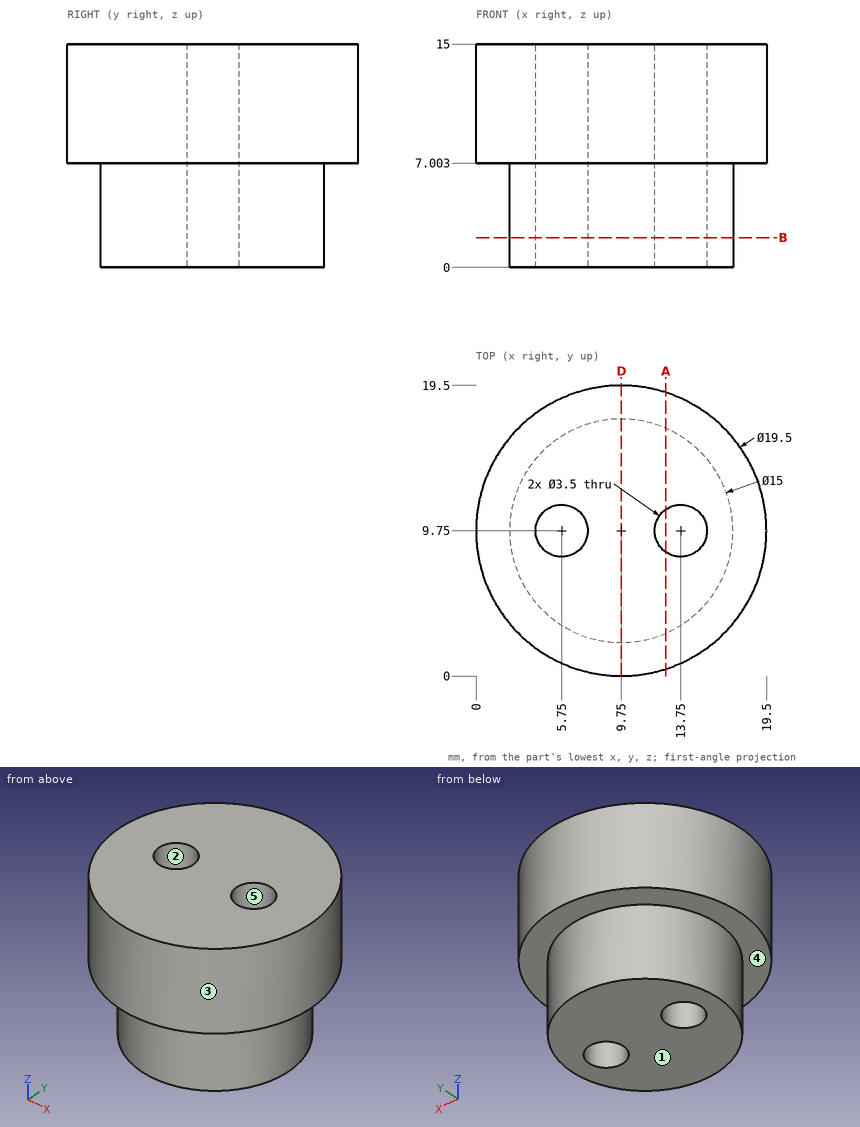
Here's the drawing with two shaded views (mm, measured from the low corner). I have some questions. A direction names the side the tool comes from. Round coordinates to 2 decimals unless told otherwise and drop trailing zeros. Loops run counter-clockwise (first coordinate to the right, second up) from the corner with the lowest first, then second, coordinate; pieces in that order, holes last.
Item 1: Suppose I cut it at A-A, the plane x = 12.75. Write out the boundary of the cut face in (y, z), then the cut area to 3 significant figures.
Item 2: Suppose I cut it at D-D, the plane x = 9.75. Write out the boundary of the cut face in (y, z).
Item 3: Will these pins go through, and if not, where does the flat tip stop? pin 1 Ø5 at (x, z) = (10.5, 13) entering from +Y; pin 2 Ø4 at (y, z) = (2, 4.5) entering from -X (1 decimal); pin 3 Ø2 at (x, y) = (16, 16) entering from -Z; pin 4 Ø1.5 at (x, z) = (9.5, 2.5) entering from -Y.
Item 4: Suppose I cut it at B-B, the plane z = 2. Write out the boundary of the cut face in (x, y).
Item 5: If we mould it in two halves opening along X, with no side actions, what happens to the marked faces 1, 2 and 3? For each: +X half, -X half, draft (parallel to the pull), parting line (faces both ways), or undercut.
Item 6: Which directions (+Z, -Z, +X, -X, +Y, -Y) give clear straight access to the entire face, cutting with the end or side of a thin tool? Please do the marked faces 4 and 5.
Item 7: Please list where these lines run through material, in increasing order: L1, parallel to Y at x = 13.75, z = 11.5; L2, parallel to X at y = 10.25, z = 7.75; L3, parallel to Z at x = 17, y = 15.
Reported:
1. outline: (0.47, 7) - (2.88, 7) - (2.88, 0) - (8.31, 0) - (8.31, 15) - (0.47, 15) - close; (11.19, 0) - (16.62, 0) - (16.62, 7) - (19.03, 7) - (19.03, 15) - (11.19, 15) - close
1. area: 202 mm2
2. outline: (0, 7) - (2.25, 7) - (2.25, 0) - (17.25, 0) - (17.25, 7) - (19.5, 7) - (19.5, 15) - (0, 15) - close
3. pin 1: stops at y = 19.5
3. pin 2: stops at x = 4.9
3. pin 3: stops at z = 7
3. pin 4: stops at y = 2.25
4. outline: circle Ø15 at (9.75, 9.75); hole circle Ø3.5 at (5.75, 9.75); hole circle Ø3.5 at (13.75, 9.75)
5. face 1: draft
5. face 2: undercut
5. face 3: parting line
6. face 4: -Z
6. face 5: +Z, -Z
7. L1: y = 0.86 to 8, 11.5 to 18.64
7. L2: x = 0.01 to 4.07, 7.43 to 12.07, 15.43 to 19.49
7. L3: z = 7 to 15
